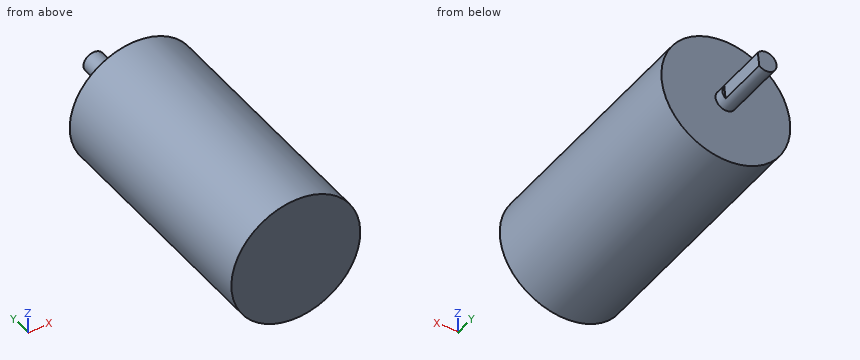
from build123d import *

# Parameters (mm, degrees)
SKETCH_1_R          = 12.5
EXTRUDE_1_DEPTH     = 48
SKETCH_2_R          = 2
EXTRUDE_2_DEPTH     = 12
CUT_EXTRUDE_START   = -10
CUT_EXTRUDE_1_DEPTH = 10


with BuildPart() as part:
    # 草图1 → 凸台-拉伸1 (new body)
    with BuildSketch(Plane(origin=(0, 0, 0), x_dir=(1, 0, 0), z_dir=(0, 1, 0))):
        with Locations(Location((0, 0, 0), (0, 0, 270))):
            Circle(SKETCH_1_R)
    extrude(amount=EXTRUDE_1_DEPTH)

    # 草图2 → 凸台-拉伸2 (add)
    with BuildSketch(Plane(origin=(0, 48, 0), x_dir=(1, 0, 0), z_dir=(0, 1, 0))):
        with Locations(Location((0, 0, 0), (0, 0, 270))):
            Circle(SKETCH_2_R)
    extrude(amount=EXTRUDE_2_DEPTH)

    # 草图3 → 切除-拉伸1 (cut)
    with BuildSketch(Plane(origin=(0, 60, 0), x_dir=(1, 0, 0), z_dir=(0, 1, 0)).offset(CUT_EXTRUDE_START)):
        with BuildLine():
            Line((1.62898558, -1.160347353), (1.354869647, 1.471165606))
            ThreePointArc((1.354869647, 1.471165606), (1.989236818, 0.207212169), (1.62898558, -1.160347353))
        make_face()
    extrude(amount=CUT_EXTRUDE_1_DEPTH, mode=Mode.SUBTRACT)


solid = part.part
CAD build for the part. Positions are in the model's coordinates, mm. Coordinates: 2 decimals unless noted, no trailing zeros. Loops run counter-clockwise (first coordinate to the right, second up) from the corner with the lowest first, then second, coordinate; pieces in that order, holes last. Notation, with made-up numbers: (19, -1.75) - (42, -1.75) arc R19 ccw to (42, 7.25) - close; hole circle Ø11 at (-35, 12.25). An arc over 180 degrees is marked (long way). Use one line per item in the form item = value. Start each with the question number.
1) Band-saw the part on C-C (y = 55). Give the cut face in (x, z).
2) Flat gauge pins, fed straight in: pin 1 (8 mm diameter, centred on x = 5.5, y = 11.5, fed in from -Z); pin 2 (8 mm diameter, centred on x = -7.5, z = -7, fed in from +Y); pin 3 (2 mm diameter, centred on y = 47.5, z = -3.5, fed in from +X). Where does each tip first touch, or does it go through?
3) Drill centre lines: L1, parallel to Y at x = -1, z = 10.5; L2, parallel to X at y = 18, z = -0.5. Where is each one in solid material? Low to high. Write a range as from..to.
4) Band-saw the part on B-B (z = 0). Give the cut face in (x, y), and give its area (3 significant figures).
5) Band-saw the part on D-D (x = -3.5). Give the cut face in (y, z).
6) Band-saw the part on A-A (x = 0). Give the cut face in (y, z), and give its area (3 significant figures).
Check values:
q1.outline = (1.35, -1.47) - (1.63, 1.16) arc R2 ccw (long way) to start
q2.pin_1 = -12.41
q2.pin_2 = 48
q2.pin_3 = 12.25
q3.L1 = 0..48
q3.L2 = -12.49..12.49
q4.outline = (-12.5, 0) - (12.5, 0) - (12.5, 48) - (2, 48) - (2, 50) - (1.51, 50) - (1.51, 60) - (-2, 60) - (-2, 48) - (-12.5, 48) - close
q4.area = 1,240 mm2
q5.outline = (0, -12) - (48, -12) - (48, 12) - (0, 12) - close
q6.outline = (0, -12.5) - (48, -12.5) - (48, -2) - (60, -2) - (60, 2) - (48, 2) - (48, 12.5) - (0, 12.5) - close
q6.area = 1,250 mm2
